Job drawing, mm, ordinate dimensions from the low corner. One solid piece. Coordinates: 2 decimals unless noted, no trailing zeros. Write each loop counter-clockwise with the first axis right and the second up, starting at its lowest first coordinate (ties: lowest second). Pieces come first, ordered by that corner, then holes. Notation, with made-up numbers: (23, 4.25) - (79, 4.25) arc R21 ccw to (79, 24.25) - close; hole circle Ø7 at (7.25, 29). An arc over 180 degrees is marked (long way). Put each result on its own line as item: value. Start each with the question number.
1. Saw through at C-C, the plane z = 1.7. Give the number of separate pieces and of enclosed holes in the cut face, plus the area to 3 significant figures.
2. Drill centre lines: L1, parallel to Y at x = 52.5, z = 1.85; L2, parallel to Y at x = 19, z = 0.55; L3, parallel to X at y = 15, z = 1.15 (1 decimal). Where is each one in solid material? Low to high. Write a range as from..to.
3. Saw through at A-A, the plane x = 50.5. Write the cut outline in (y, z).
4. Drop a flat-ended pin along its axis: P1, Ø1, axis at y = 14, z = 1, coming from the -X side. Give the stop position or say it passes through.
5. Saw through at D-D, the plane x = 11. Write the cut outline in (y, z).
6. Saw through at B-B, the plane y = 11.5. Write the cut outline in (x, z) (1 decimal).
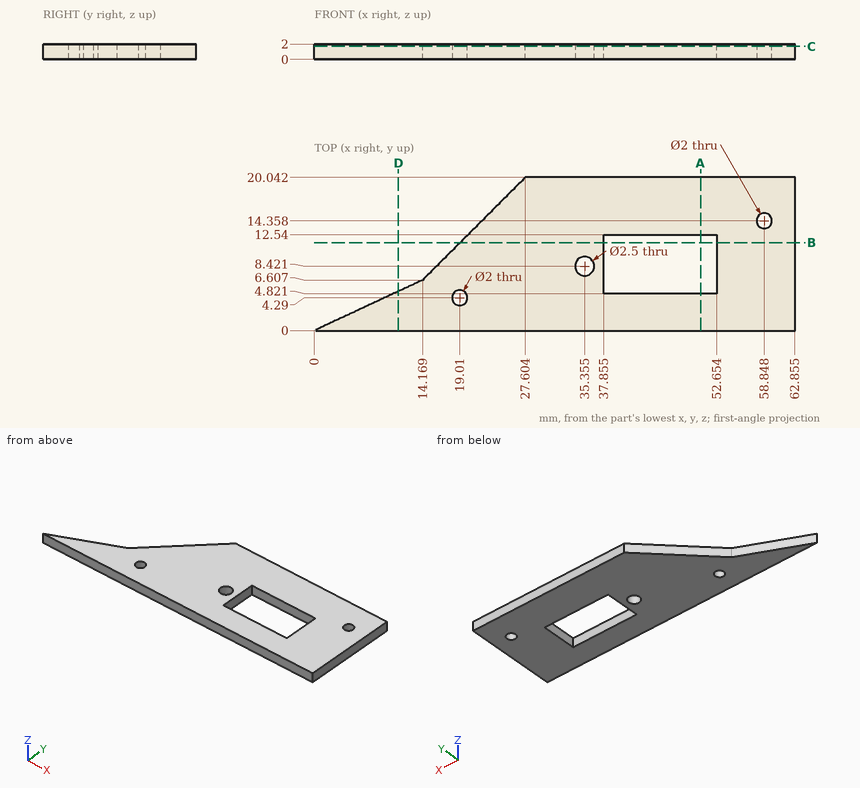
Final values:
1. separate pieces: 1
1. enclosed holes: 4
1. area: 807 mm²
2. L1: y = 0..4.82, 12.54..20.04
2. L2: y = 0..3.29, 5.29..11.44
2. L3: x = 22.6..58.1, 59.6..62.9
3. outline: (0, 0) - (4.82, 0) - (4.82, 2) - (0, 2) - close; (12.54, 0) - (20.04, 0) - (20.04, 2) - (12.54, 2) - close
4. P1: stops at x = 21.06
5. outline: (0, 0) - (5.13, 0) - (5.13, 2) - (0, 2) - close
6. outline: (19.1, 0) - (37.9, 0) - (37.9, 2) - (19.1, 2) - close; (52.7, 0) - (62.9, 0) - (62.9, 2) - (52.7, 2) - close
